```python
from build123d import *

# Parameters (mm, degrees)
CROQUIS1_W              = 195
CROQUIS1_H              = 38
CROQUIS1_R              = 1.625
SALIENTE_EXTRUIR1_DEPTH = 3
SALIENTE_EXTRUIR2_START = -67.5
SALIENTE_EXTRUIR2_DEPTH = 45
SALIENTE_EXTRUIR3_START = -67.5
SALIENTE_EXTRUIR3_DEPTH = 45
CROQUIS8_W              = 195
CROQUIS8_H              = 3
SALIENTE_EXTRUIR5_DEPTH = 5
CROQUIS9_R              = 8.25
CORTAR_EXTRUIR4_DEPTH   = 106.640382748
CROQUIS10_W             = 195
CROQUIS10_H             = 3
SALIENTE_EXTRUIR6_DEPTH = 15
CORTAR_EXTRUIR5_DEPTH   = 15


with BuildPart() as part:
    # Croquis1 → Saliente-Extruir1 (new body)
    with BuildSketch(Plane.XY):
        with Locations((0, 19)):
            Rectangle(CROQUIS1_W, CROQUIS1_H)
        with Locations((91.125, 15)):
            Circle(CROQUIS1_R, mode=Mode.SUBTRACT)
        with Locations(Location((-91.125, 15, 0), (0, 0, 180))):
            Circle(CROQUIS1_R, mode=Mode.SUBTRACT)
    extrude(amount=SALIENTE_EXTRUIR1_DEPTH)

    # Croquis2 → Saliente-Extruir2 (add)
    with BuildSketch(Plane(origin=(97.5, 0, 0), x_dir=(0, 0, -1), z_dir=(1, 0, 0)).offset(SALIENTE_EXTRUIR2_START)):
        Polygon((0, 0.738403157), (3.429565646, 3.677896428), (15.185426147, 13.753887502), (0, 31.471028189), align=None)
    extrude(amount=SALIENTE_EXTRUIR2_DEPTH)

    # Croquis4 → Saliente-Extruir3 (add)
    with BuildSketch(Plane.ZY.offset(97.5).offset(SALIENTE_EXTRUIR3_START)):
        Polygon((0, 0.738403157), (-15.185426147, 13.753887502), (0, 31.471028189), align=None)
    extrude(amount=SALIENTE_EXTRUIR3_DEPTH)

    # Croquis8 → Saliente-Extruir5 (add)
    with BuildSketch(Plane.XZ):
        with Locations((0, 1.5)):
            Rectangle(CROQUIS8_W, CROQUIS8_H)
    extrude(amount=SALIENTE_EXTRUIR5_DEPTH)

    # Croquis9 → Cortar-Extruir4 (cut, through all)
    with BuildSketch(Plane(origin=(0, 0.425684191, 0.364855478), x_dir=(1, 0, 0), z_dir=(0, -0.7592713073348798, -0.6507742172658522))):
        with Locations(Location((-65.42, -10.480533736, 0), (0, 0, 270))):
            Circle(CROQUIS9_R)
        with Locations(Location((-39.57, -10.480533736, 0), (0, 0, 270))):
            Circle(CROQUIS9_R)
        with Locations(Location((39.57, -10.480533736, 0), (0, 0, 90))):
            Circle(CROQUIS9_R)
        with Locations(Location((65.42, -10.480533736, 0), (0, 0, 90))):
            Circle(CROQUIS9_R)
    extrude(amount=-CORTAR_EXTRUIR4_DEPTH, mode=Mode.SUBTRACT)

    # Croquis10 → Saliente-Extruir6 (add)
    with BuildSketch(Plane(origin=(0, 38, 0), x_dir=(1, 0, 0), z_dir=(0, 1, 0))):
        with Locations((0, -1.5)):
            Rectangle(CROQUIS10_W, CROQUIS10_H)
    extrude(amount=SALIENTE_EXTRUIR6_DEPTH)

    # Croquis11 → Cortar-Extruir5 (cut)
    with BuildSketch(Plane(origin=(0, 0, 0), x_dir=(-1, 0, 0), z_dir=(0, 0, -1))):
        with BuildLine():
            Line((-92.75, 15), (-92.75, 35))
            ThreePointArc((-92.75, 35), (-91.125, 36.625), (-89.5, 35))
            Line((-89.5, 35), (-89.5, 15))
            ThreePointArc((-89.5, 15), (-91.125, 13.375), (-92.75, 15))
        make_face()
        with BuildLine():
            Line((89.5, 35), (89.5, 15))
            ThreePointArc((89.5, 15), (91.125, 13.375), (92.75, 15))
            Line((92.75, 15), (92.75, 35))
            ThreePointArc((92.75, 35), (91.125, 36.625), (89.5, 35))
        make_face()
    extrude(amount=-CORTAR_EXTRUIR5_DEPTH, mode=Mode.SUBTRACT)


solid = part.part
```
Build history of the part. All positions in model axes, mm. A direction names the side the tool comes from. Coordinates: 2 decimals unless noted, no trailing zeros. Order: outer loops, then holes, each group sorted by start corner. A loop starts at its lowest first (then second) coordinate and runs counter-clockwise, first axis right, second up. Notation, with made-up numbers: (72.25, 73) -> (124.25, 73) arc R20 ccw to (124.25, 107) -> close; hole circle Ø5 at (-16, -2). An arc over 180 degrees is marked (long way). Answer in a Markdown table with one row per item. Add a question column.
Q1. Which spindle directions (+Z, -Z, +X, -X, +Y, -Y) get a long thin tool onto all of the face, cutting with end or side? Do faces 5 (the face through (-75, 16, -4)), 6 (the face through (-37.09, 19.88, -7.13)), 7 (the face through (30, 16, -4)). Say none if no direction does.
Q2. Band-saw the part on C-C, the plane y = 23.5. Give the number of separate pieces and of enclosed holes in the cut face, then the cut area to 3 significant figures.
Q3. Drop flat-ended pins along their axis: pin 1 (4.5 mm diameter, centred on y = 23, z = -7.5, fed in from +X); pin 2 (12 mm diameter, centred on x = -43.5, y = 39, fed in from -Z); pin 3 (7.5 mm diameter, centred on y = 15.5, z = -9, fed in from -X); pin 4 (2 mm diameter, centred on x = 10, z = -2, fed in from -Y). Give the stop position or say it passes through.
Q4. Wall check: line 1 along X through (y, z) = (13, -4.75); line 2 along X through (y, z) = (10, -6.75); line 3 along Z through (x, y) = (79, 14.5). Give the ranges that are in metal, low to high. Write a range as [from, to].
Q5. Band-saw the part on A-A, the plane y = 48. List the corners of the cut face in (x, z), then the cut area to 3 significant figures.
Q6. Band-saw the part on B-B, the plane x = 80. List the corners of the cut face in (y, z), then the cut area to 3 significant figures.
Q7. Mould opens along Z. For faces 1 (the face through (65.06, 20.24, -7.31)), 2 (the face through (-62.94, 19.88, -7.13)), 3 (the face through (52.18, 22.49, -7.7)), 4 (the face through (75, 16, -4)) say: +Z half, -Z half, draft (parallel to the pull), parting line (faces both ways), or undercut.
Answers follow:
| question | item | result |
|---|---|---|
| 1 | face 5 | -Z, -X, +Y, -Y |
| 1 | face 6 | none |
| 1 | face 7 | -Z, +Y, -Y |
| 2 | separate pieces | 3 |
| 2 | enclosed holes | 0 |
| 2 | area | 834 mm^2 |
| 3 | pin 1 | x = 75 |
| 3 | pin 2 | z = 0 |
| 3 | pin 3 | x = -75 |
| 3 | pin 4 | through |
| 4 | line 1 | [-75, -73.52], [-57.32, -47.67], [-31.47, -30], [30, 31.47], [47.67, 57.32], [73.52, 75] |
| 4 | line 2 | [-75, -73.59], [-57.25, -47.74], [-31.4, -30], [30, 31.4], [47.74, 57.25], [73.59, 75] |
| 4 | line 3 | [0, 3] |
| 5 | outline | (-97.5, 0) -> (97.5, 0) -> (97.5, 3) -> (-97.5, 3) -> close |
| 5 | area | 585 mm^2 |
| 6 | outline | (-5, 0) -> (53, 0) -> (53, 3) -> (-5, 3) -> close |
| 6 | area | 174 mm^2 |
| 7 | face 1 | undercut |
| 7 | face 2 | undercut |
| 7 | face 3 | -Z half |
| 7 | face 4 | draft |
